```python
from build123d import *

# Parameters (mm, degrees)
SKETCH1_R              = 55
SKETCH1_R_2            = 3
BOSS_EXTRUDE1_DEPTH    = 39.9
SKETCH2_R              = 52
CUT_EXTRUDE1_DEPTH     = 60
CUT_EXTRUDE2_START     = -39.9
CUT_EXTRUDE2_OUTLINE_R = 3
CUT_EXTRUDE2_DEPTH     = 39.9
EXTRUDE_THIN1_START    = -10
SKETCH4_R              = 59
SKETCH4_R_2            = 55
EXTRUDE_THIN1_DEPTH    = 30
FILLET1_R              = 10
FILLET2_R              = 10


# Read off the part's stored shape, not the designer's step: Cut-Extrude2
with BuildPart() as part:
    # Sketch1 → Boss-Extrude1 (new body)
    with BuildSketch(Plane.XY):
        Circle(SKETCH1_R)
        Circle(SKETCH1_R_2, mode=Mode.SUBTRACT)
    extrude(amount=BOSS_EXTRUDE1_DEPTH)

    # Sketch2 → Cut-Extrude1 (cut)
    with BuildSketch(Plane.XY.offset(39.9)):
        Circle(SKETCH2_R)
        with BuildLine():
            Line((-41.361950208, 16.620711788), (-41.361950208, -16.620711788))
            ThreePointArc((-41.361950208, -16.620711788), (0, -44.576439802), (41.361950208, -16.620711788))
            Line((41.361950208, -16.620711788), (41.361950208, 16.620711788))
            ThreePointArc((41.361950208, 16.620711788), (0, 44.576439802), (-41.361950208, 16.620711788))
        make_face(mode=Mode.SUBTRACT)
    extrude(amount=-CUT_EXTRUDE1_DEPTH, mode=Mode.SUBTRACT)


with BuildPart() as cut_extrude1_piece_1:
    # of the separate pieces the step leaves, piece 1, a body of its own (cut_extrude1_pieces)
    add(part.part.solids().sort_by_distance((41.361950208, -16.620711788, 0))[0])

    # Cut-Extrude2 outline → Cut-Extrude2 (cut)
    with BuildSketch(Plane.XY.offset(39.9).offset(CUT_EXTRUDE2_START)):
        with BuildLine():
            Line((41.361950208, -16.620711788), (41.361950208, 16.620711788))
            ThreePointArc((41.361950208, 16.620711788), (0, 44.576439802), (-41.361950208, 16.620711788))
            Line((-41.361950208, 16.620711788), (-41.361950208, -16.620711788))
            ThreePointArc((-41.361950208, -16.620711788), (0, -44.576439802), (41.361950208, -16.620711788))
        make_face()
        Circle(CUT_EXTRUDE2_OUTLINE_R, mode=Mode.SUBTRACT)
    extrude(amount=CUT_EXTRUDE2_DEPTH, mode=Mode.SUBTRACT)


with BuildPart() as cut_extrude1_piece_2:
    # of the separate pieces the step leaves, piece 2, a body of its own (cut_extrude1_pieces)
    add(part.part.solids().sort_by_distance((55, 0, 0))[0])

    # Sketch4 → Extrude-Thin1 (add)
    with BuildSketch(Plane.XY.offset(39.9).offset(EXTRUDE_THIN1_START)):
        Circle(SKETCH4_R)
        Circle(SKETCH4_R_2, mode=Mode.SUBTRACT)
    extrude(amount=EXTRUDE_THIN1_DEPTH)

    # Fillet1
    # the kernel refuses this fillet: 10 mm, written as the material it adds along each edge
    with BuildSketch(Plane(origin=(0, 0, 29.9), x_dir=(1, 0, 0), z_dir=(0, -1, 0))) as fillet1_piece_1:
        with BuildLine():
            CenterArc((65, -8), FILLET1_R, 126.869897646, 53.130102354)
            Line((59, 0), (58.88, 0.16))
            ThreePointArc((58.88, 0.16), (57, 0.2), (55, 0.2))
            Line((55, 0.2), (54.8, 0))
            Line((54.8, 0), (54.8, -8))
            Line((54.8, -8), (55, -8))
        make_face()
    revolve(axis=Axis((0, 0, 29.9), (0, 0, 1)))

    # Fillet2
    # the kernel refuses this fillet: 10 mm, written as the material it adds along each edge
    with BuildSketch(Plane(origin=(0, 0, 39.9), x_dir=(1, 0, 0), z_dir=(0, -1, 0))) as fillet2_piece_1:
        with BuildLine():
            CenterArc((45, 7.141428429), FILLET2_R, 314.427004001, 45.572995999)
            Line((52, 0), (52.14, -0.142828569))
            ThreePointArc((52.14, -0.142828569), (53.5, -0.2), (55, -0.2))
            Line((55, -0.2), (55.2, 0))
            Line((55.2, 0), (55.2, 7.141428429))
            Line((55.2, 7.141428429), (55, 7.141428429))
        make_face()
    revolve(axis=Axis((0, 0, 39.9), (0, 0, 1)))


solid = cut_extrude1_piece_2.part
```
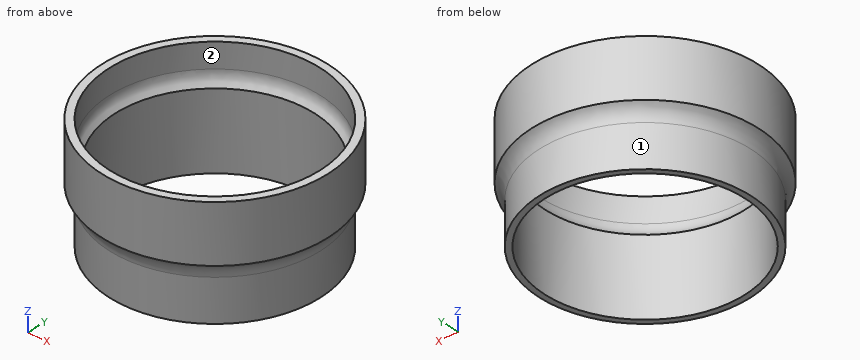
Geometry check sheet. Reference: the model listing, model coordinates, mm. Face numbers are marked on the shaded views. Round coordinates to 2 decimals unless told otherwise and drop trailing zeros. Write each loop counter-clockwise with the first axis right and the second up, starting at its lowest first coordinate (ties: lowest second). Pieces come first, ordered by that corner, then holes. Notation, with made-up numbers: (-17.5, 12.25) - (20.5, 12.25) arc R25 ccw to (20.5, 32.25) - close; hole circle Ø8 at (-28, 58). An arc over 180 degrees is marked (long way). Write each question's results on one line, items separated by ' | '.
(1) Sectioned sample at C-C, the plane z = 18. Enter the section's corners in (x, y).
Computed:
outline: circle Ø110 at (0, 0); hole circle Ø104 at (0, 0)
(2) Sectioned sample at A-A, the plane x = 0. Enter the section's corners in (y, z), plus the area to 3 significant figures.
Computed:
outline: (-59, 29.9) arc R10 cw to (-55, 21.9) - (-55, 0) - (-52, 0) - (-52, 39.9) arc R10 cw to (-55, 47.04) - (-55, 59.9) - (-59, 59.9) - close; (52, 0) - (55, 0) - (55, 21.9) arc R10 cw to (59, 29.9) - (59, 59.9) - (55, 59.9) - (55, 47.04) arc R10 cw to (52, 39.9) - close | area: 512 mm^2
(3) Thickness scan on probe 1 along Y at (x, z) = (0, 50.75); probe 2 along Y at (x, z) = (0, 19); probe 3 along X at (y, z) = (-42, 42). Record the ranges inside material, lowest first. Write a range as from..to.
Computed:
probe 1: y = -59..-55, 55..59 | probe 2: y = -55..-52, 52..55 | probe 3: x = -41.44..-33.36, 33.36..41.44
(4) Depth check by flat-ended pin: pin 1 Ø3 at (x, z) = (-41.5, 36.5) entering from +Y; pin 2 Ø8 at (y, z) = (14, 15.5) entering from -X; pin 3 Ø1 at (x, y) = (-36, 36) entering from +Z; pin 4 Ø1 at (x, z) = (-28.5, 47.5) entering from +Y. Enter the tip coordinate at first touch or a pass-through.
Computed:
pin 1: stops at y = 43.37 | pin 2: stops at x = -54.08 | pin 3: passes through | pin 4: stops at y = 51.93
(5) Draft check along Y on the marked faces 1 and 2. Enter one of: pulls with the +Y half, pulls with the -Y half, needs draft (parallel to the pull), parting line crosses it, or undercut.
Computed:
face 1: parting line crosses it | face 2: undercut
